Model file for the job. Use its own axes, mm. A direction names the side the tool comes from. Coordinates: 2 decimals unless noted, no trailing zeros. Write each loop counter-clockwise with the first axis right and the second up, starting at its lowest first coordinate (ties: lowest second). Pieces come first, ordered by that corner, then holes. Notation, with made-up numbers: (44.5, -8.75) - (74.5, -8.75) arc R20 ccw to (74.5, 27.25) - close; hole circle Ø6 at (-29, -16.75). An arc over 180 degrees is marked (long way). Put each result on its own line as item: value. Start each with the question number.
1. Saw through at B-B, the plane y = 2.15. Write the cut outline in (x, z).
2. Saw through at D-D, the plane z = -8.5. Write the cut outline in (x, y), plus the area to 3 significant figures.
3. Which spindle directions (+Z, -Z, +X, -X, +Y, -Y) get a long thin tool onto all of the face, cutting with end or side? Do faces 5 (the face through (90, 1, -2)), 6 (the face through (62, 1, -10)), 7 (the face through (150, 1, -11)), 8 (the face through (-2, 1, -5)). Say none if no direction does.
4. Saw through at A-A, the plane z = -1.75. Write the cut outline in (x, y).
5. Drill centre lines: L1, parallel to X at y = 2.05, z = -12; L2, parallel to X at y = 1.4, z = -0.5; L3, parallel to Z at x = 7, y = 2.25. Where is each one in solid material? Low to high. Write a range as from..to.
6. Drop flat-ended pins along their axis: P1, Ø1.5, axis at y = 2, z = -8.5, coming from the +X side; P2, Ø1.5, axis at x = -2, y = 1, coming from the -Z side; P3, Ø1, axis at y = 0.5, z = -11.5, coming from the -X side. Give the stop position or say it passes through.
7. Saw through at C-C, the plane x = 69. Write the cut outline in (y, z).
8. Pull direction X, two halves, no side cores. Call faces 1 (the face through (37, 1, -13)), 2 (the face through (25, 1, -11)), 3 (the face through (112, 1, -10)), 4 (the face through (125, 1, -11)): released by +X, released by -X, zero draft, split by the parting line, or undercut.
```python
from build123d import *

# Parameters (mm, degrees)
SKICA1_W                 = 175
SKICA1_H                 = 10
P_IDAT_VYSUNUT_M1_DEPTH  = 3
SKICA2_W                 = 3
SKICA2_H                 = 5
SKICA2_W_2               = 25
SKICA2_H_2               = 3
P_IDAT_VYSUNUT_M2_DEPTH  = 3
SKICA3_W                 = 3
SKICA3_H                 = 5
ODEBRAT_VYSUNUT_M1_DEPTH = 179.499299719


with BuildPart() as part:
    # Skica1 → Přidat vysunutím1 (new body)
    with BuildSketch(Plane(origin=(0, 0, 0), x_dir=(1, 0, 0), z_dir=(0, 1, 0))):
        with Locations((87.5, 5)):
            Rectangle(SKICA1_W, SKICA1_H)
    extrude(amount=P_IDAT_VYSUNUT_M1_DEPTH)

    # Skica2 → Přidat vysunutím2 (add)
    with BuildSketch(Plane(origin=(0, 0, 0), x_dir=(1, 0, 0), z_dir=(0, 1, 0))):
        with Locations((-1.5, 2.5)):
            Rectangle(SKICA2_W, SKICA2_H)
        with Locations((176.5, 2.5)):
            Rectangle(SKICA2_W, SKICA2_H)
        with Locations((37.5, 11.5)):
            Rectangle(SKICA2_W_2, SKICA2_H_2)
        with Locations((87.5, 11.5)):
            Rectangle(SKICA2_W_2, SKICA2_H_2)
        with Locations((137.5, 11.5)):
            Rectangle(SKICA2_W_2, SKICA2_H_2)
    extrude(amount=P_IDAT_VYSUNUT_M2_DEPTH)

    # Skica3 → Odebrat vysunutím1 (cut, through all)
    with BuildSketch(Plane(origin=(0, 0, 0), x_dir=(1, 0, 0), z_dir=(0, 1, 0))):
        with Locations((88.5, 2.5)):
            Rectangle(SKICA3_W, SKICA3_H)
    extrude(amount=ODEBRAT_VYSUNUT_M1_DEPTH, mode=Mode.SUBTRACT)


solid = part.part
```
Final values:
1. outline: (-3, -5) - (0, -5) - (0, -10) - (25, -10) - (25, -13) - (50, -13) - (50, -10) - (75, -10) - (75, -13) - (100, -13) - (100, -10) - (125, -10) - (125, -13) - (150, -13) - (150, -10) - (175, -10) - (175, -5) - (178, -5) - (178, 0) - (90, 0) - (90, -5) - (87, -5) - (87, 0) - (-3, 0) - close
2. outline: (0, 0) - (175, 0) - (175, 3) - (0, 3) - close
2. area: 525 mm²
3. face 5: +Z, +Y, -Y
3. face 6: -Z, +Y, -Y
3. face 7: -Z, +X, +Y, -Y
3. face 8: -Z, -X, +Y, -Y
4. outline: (-3, 0) - (87, 0) - (87, 3) - (-3, 3) - close; (90, 0) - (178, 0) - (178, 3) - (90, 3) - close
5. L1: x = 25..50, 75..100, 125..150
5. L2: x = -3..87, 90..178
5. L3: z = -10..0
6. P1: stops at x = 175
6. P2: stops at z = -5
6. P3: stops at x = 25
7. outline: (0, -10) - (3, -10) - (3, 0) - (0, 0) - close
8. face 1: zero draft
8. face 2: released by -X
8. face 3: undercut
8. face 4: undercut
